The listing builds one solid part. Answer for the finished solid, in the listing's coordinates (mm). A direction names the side the tool comes from. Give positions to 0.01 mm unless a question says otherwise; leave off trailing zeros. Order: outer loops, then holes, each group sorted by start corner. A loop starts at its lowest first (then second) coordinate and runs counter-clockwise, first axis right, second up. Notation, with made-up numbers: (24.5, 59.25) -> (71.5, 59.25) arc R33 cw to (71.5, 87.25) -> close; hole circle Ø1 at (11.5, -1). An arc over 180 degrees is marked (long way). One line per question, with ' | ' between items. Start each with the question number.
```python
from build123d import *

# Parameters (mm, degrees)
SKETCH1_R           = 5
BOSS_EXTRUDE2_DEPTH = 10
CUT_EXTRUDE1_DEPTH  = 25
SKETCH4_R           = 2.5
CUT_EXTRUDE2_DEPTH  = 38


with BuildPart() as part:
    # Sketch1 → Boss-Extrude2 (new body)
    with BuildSketch(Plane.XY):
        with BuildLine():
            Line((35, 15), (13.114987511, 67.279910892))
            ThreePointArc((13.114987511, 67.279910892), (0, 75), (-13.114987511, 67.279910892))
            Line((-13.114987511, 67.279910892), (-35, 15))
            Line((-35, 15), (-50, 15))
            Line((-50, 15), (-50, 0))
            Line((-50, 0), (-35, 0))
            Line((-35, 0), (35, 0))
            Line((35, 0), (50, 0))
            Line((50, 0), (50, 15))
            Line((50, 15), (35, 15))
        make_face()
        with Locations((0, 59.06)):
            Circle(SKETCH1_R, mode=Mode.SUBTRACT)
    extrude(amount=BOSS_EXTRUDE2_DEPTH)

    # Sketch3 → Cut-Extrude1 (cut)
    with BuildSketch(Plane(origin=(0, 0, 0), x_dir=(-1, 0, 0), z_dir=(0, 0, -1))):
        with BuildLine():
            Line((0, 15), (-8.596117968, 15))
            ThreePointArc((-8.596117968, 15), (-12.537145158, 16.922938953), (-13.446830469, 21.212678125))
            Line((-13.446830469, 21.212678125), (-8.446830469, 41.212678125))
            ThreePointArc((-8.446830469, 41.212678125), (-6.673179015, 43.94102719), (-3.596117968, 45))
            Line((-3.596117968, 45), (0, 45))
            Line((0, 45), (3.596117968, 45))
            ThreePointArc((3.596117968, 45), (6.673179015, 43.94102719), (8.446830469, 41.212678125))
            Line((8.446830469, 41.212678125), (13.446830469, 21.212678125))
            ThreePointArc((13.446830469, 21.212678125), (12.537145158, 16.922938953), (8.596117968, 15))
            Line((8.596117968, 15), (0, 15))
        make_face()
    extrude(amount=-CUT_EXTRUDE1_DEPTH, mode=Mode.SUBTRACT)

    # Sketch4 → Cut-Extrude2 (cut)
    with BuildSketch(Plane(origin=(0, 15, 0), x_dir=(1, 0, 0), z_dir=(0, 1, 0))):
        with Locations(Location((-42.5, -5, 0), (0, 0, 270))):
            Circle(SKETCH4_R)
        with Locations(Location((42.5, -5, 0), (0, 0, 180))):
            Circle(SKETCH4_R)
    extrude(amount=-CUT_EXTRUDE2_DEPTH, mode=Mode.SUBTRACT)


solid = part.part
```
(1) For faces 5 (the face through (0, 45, 5)), 6 (the face through (50, 7, 5)), 7 (the face through (44.3, 15, 2.7)), determine the directions among +Z, -Z, +X, -X, +Y, -Y from which every point of the face is accessible in a straight line to the end or side of a thin tool.
(2) The part is cut by section D-D on y = 62.5. Determine the outline of the cut face in (x, z).
(3) Determine the mould class of faces 1 (the face through (-11, 31, 5)), 2 (the face through (24.2, 40.8, 4.9)), 3 (the face through (-12.576, 16.973, 4.93)), 4 (the face through (-23.904, 41.506, 4.93)) for opening direction X: pulls with the +X half, pulls with the -X half, needs draft (parallel to the pull), parting line crosses it, or undercut.
(4) Given P1, Ø2, axis at y = 29.5, z = 5, coming from the +X side; P2, Ø2, axis at y = 40.5, z = 3, coming from the +X side; P3, Ø3, axis at y = 18.5, z = 8.5, coming from the -X side, each flat-ended and moving along its own axis, determine where each tip first touches the part or whether it passes through.
(5) Consider line 1 (Y direction, x = 0, z = 4.5); line 2 (Y direction, x = 7.5, z = 5.75); line 3 (Y direction, x = 3, z = 9.25). Determine where each line is inside the solid, lowest interval first.
(6) The part is cut by section B-B on x = -42.5. Determine the outline of the cut face in (y, z).
(7) The part is cut by section C-C on x = 0. Determine the outline of the cut face in (y, z).
(8) The part is cut by section A-A on z = 5. Determine the outline of the cut face in (x, y), plus the area to 3 significant figures.
Result sheet:
1) face 5: +Z, -Z | face 6: +Z, -Z, +X, +Y, -Y | face 7: +Z, -Z, +X, +Y
2) outline: (-15.12, 0) -> (-3.63, 0) -> (-3.63, 10) -> (-15.12, 10) -> close; (3.63, 0) -> (15.12, 0) -> (15.12, 10) -> (3.63, 10) -> close
3) face 1: undercut | face 2: pulls with the +X half | face 3: undercut | face 4: pulls with the -X half
4) P1: stops at x = 29.35 | P2: stops at x = 24.74 | P3: stops at x = -34.16
5) line 1: y = 0 to 15, 45 to 54.06, 64.06 to 75 | line 2: y = 0 to 15, 43.12 to 72.99 | line 3: y = 0 to 15, 45 to 55.06, 63.06 to 74.7
6) outline: (0, 0) -> (15, 0) -> (15, 2.5) -> (0, 2.5) -> close; (0, 7.5) -> (15, 7.5) -> (15, 10) -> (0, 10) -> close
7) outline: (0, 0) -> (15, 0) -> (15, 10) -> (0, 10) -> close; (45, 0) -> (54.06, 0) -> (54.06, 10) -> (45, 10) -> close; (64.06, 0) -> (75, 0) -> (75, 10) -> (64.06, 10) -> close
8) outline: (-50, 0) -> (-45, 0) -> (-45, 15) -> (-50, 15) -> close; (-40, 0) -> (40, 0) -> (40, 15) -> (35, 15) -> (13.11, 67.28) arc R15 ccw to (-13.11, 67.28) -> (-35, 15) -> (-40, 15) -> close; (45, 0) -> (50, 0) -> (50, 15) -> (45, 15) -> close; hole (-13.45, 21.21) arc R5 ccw to (-8.6, 15) -> (8.6, 15) arc R5 ccw to (13.45, 21.21) -> (8.45, 41.21) arc R5 ccw to (3.6, 45) -> (-3.6, 45) arc R5 ccw to (-8.45, 41.21) -> close; hole circle Ø10 at (0, 59.06) | area: 3,280 mm^2
